```python
from build123d import *

# Parameters (mm, degrees)
SKETCH1_W                  = 25.4
SKETCH1_H                  = 1498.6
BOSS_EXTRUDE1_DEPTH        = 25.4
SKETCH2_W                  = 23.114
SKETCH2_H                  = 23.114
CUT_EXTRUDE1_DEPTH         = 1499.6
M3_5_CLEARANCE_HOLE1_D     = 4.1402
M3_5_CLEARANCE_HOLE1_DEPTH = 25.4
M3_5_CLEARANCE_HOLE2_D     = 4.1402
M3_5_CLEARANCE_HOLE2_DEPTH = 25.4
CHAMFER1_SIZE              = 2.159
FILLET1_R                  = 0.8128
FILLET2_R                  = 3.0988
SKETCH8_W                  = 95.882963774
SKETCH8_H                  = 79.338329604
CUT_EXTRUDE3_DEPTH         = 1371.6
SKETCH11_W                 = 51.462522779
SKETCH11_H                 = 66.676735099
CUT_EXTRUDE6_DEPTH         = 2.286


with BuildPart() as part:
    # Sketch1 → Boss-Extrude1 (new body)
    with BuildSketch(Plane(origin=(0, 0, 0), x_dir=(0, -1, 0), z_dir=(-1, 0, 0))):
        with Locations((-12.7, 0)):
            Rectangle(SKETCH1_W, SKETCH1_H)
    extrude(amount=-BOSS_EXTRUDE1_DEPTH)

    # Sketch2 → Cut-Extrude1 (cut, through all)
    with BuildSketch(Plane(origin=(0, 0, -749.3), x_dir=(-1, 0, 0), z_dir=(0, 0, -1))):
        with Locations((-13.843, 13.843)):
            Rectangle(SKETCH2_W, SKETCH2_H)
    extrude(amount=-CUT_EXTRUDE1_DEPTH, mode=Mode.SUBTRACT)

    # M3.5 Clearance Hole1
    with Locations(Plane(origin=(0, 0, 0), x_dir=(-1, 0, 0), z_dir=(0, -1, 0))):
        with Locations((-12.7, 736.6), (-12.7, 711.2), (-12.7, 685.8), (-12.7, 660.4), (-12.7, 635), (-12.7, 609.6), (-12.7, 584.2), (-12.7, 558.8), (-12.7, 533.4), (-12.7, 508), (-12.7, 482.6), (-12.7, 457.2), (-12.7, 431.8), (-12.7, 406.4), (-12.7, 381), (-12.7, 355.6), (-12.7, 330.2), (-12.7, 304.8), (-12.7, 279.4), (-12.7, 254), (-12.7, 228.6), (-12.7, 203.2), (-12.7, 177.8), (-12.7, 152.4), (-12.7, 127), (-12.7, 101.6), (-12.7, 76.2), (-12.7, 50.8), (-12.7, 25.4), (-12.7, 0), (-12.7, -25.4), (-12.7, -50.8), (-12.7, -76.2), (-12.7, -101.6), (-12.7, -127), (-12.7, -152.4), (-12.7, -177.8), (-12.7, -203.2), (-12.7, -228.6), (-12.7, -254), (-12.7, -279.4), (-12.7, -304.8), (-12.7, -330.2), (-12.7, -355.6), (-12.7, -381), (-12.7, -406.4), (-12.7, -431.8), (-12.7, -457.2), (-12.7, -482.6), (-12.7, -508), (-12.7, -533.4), (-12.7, -558.8), (-12.7, -584.2), (-12.7, -609.6), (-12.7, -635), (-12.7, -660.4), (-12.7, -685.8), (-12.7, -711.2), (-12.7, -736.6)):
            Hole(M3_5_CLEARANCE_HOLE1_D / 2, depth=M3_5_CLEARANCE_HOLE1_DEPTH)

    # M3.5 Clearance Hole2
    with Locations(Plane.ZY):
        with Locations((711.2, 12.7), (736.6, 12.7), (685.8, 12.7), (660.4, 12.7), (635, 12.7), (609.6, 12.7), (584.2, 12.7), (558.8, 12.7), (533.4, 12.7), (508, 12.7), (482.6, 12.7), (457.2, 12.7), (431.8, 12.7), (406.4, 12.7), (381, 12.7), (355.6, 12.7), (330.2, 12.7), (304.8, 12.7), (279.4, 12.7), (254, 12.7), (228.6, 12.7), (203.2, 12.7), (177.8, 12.7), (152.4, 12.7), (127, 12.7), (101.6, 12.7), (76.2, 12.7), (50.8, 12.7), (25.4, 12.7), (0, 12.7), (-25.4, 12.7), (-50.8, 12.7), (-76.2, 12.7), (-101.6, 12.7), (-127, 12.7), (-152.4, 12.7), (-177.8, 12.7), (-203.2, 12.7), (-228.6, 12.7), (-254, 12.7), (-279.4, 12.7), (-304.8, 12.7), (-330.2, 12.7), (-355.6, 12.7), (-381, 12.7), (-406.4, 12.7), (-431.8, 12.7), (-457.2, 12.7), (-482.6, 12.7), (-508, 12.7), (-533.4, 12.7), (-558.8, 12.7), (-584.2, 12.7), (-609.6, 12.7), (-635, 12.7), (-660.4, 12.7), (-685.8, 12.7), (-711.2, 12.7), (-736.6, 12.7)):
            Hole(M3_5_CLEARANCE_HOLE2_D / 2, depth=M3_5_CLEARANCE_HOLE2_DEPTH)

    # Chamfer1
    chamfer1_edges = [part.edges().sort_by_distance(p)[0] for p in [
        (25.4, 1.143, -749.3),
        (1.143, 25.4, 749.3),
        (1.143, 25.4, -749.3),
        (25.4, 1.143, 749.3),
    ]]
    chamfer(chamfer1_edges, length=CHAMFER1_SIZE)

    # Fillet1
    fillet1_edges = [part.edges().sort_by_distance(p)[0] for p in [
        (2.286, 2.286, 0),
    ]]
    fillet(fillet1_edges, radius=FILLET1_R)

    # Fillet2
    fillet2_edges = [part.edges().sort_by_distance(p)[0] for p in [
        (0, 0, 0),
    ]]
    fillet(fillet2_edges, radius=FILLET2_R)

    # Sketch8 → Cut-Extrude3 (cut)
    with BuildSketch(Plane.XY.offset(749.3)):
        with Locations((2.286, 3.0988)):
            Rectangle(SKETCH8_W, SKETCH8_H)
    extrude(amount=-CUT_EXTRUDE3_DEPTH, mode=Mode.SUBTRACT)

    # Sketch11 → Cut-Extrude6 (cut)
    with BuildSketch(Plane.XY.offset(-622.3)):
        with Locations((1.85517497, 1.74884985)):
            Rectangle(SKETCH11_W, SKETCH11_H)
    extrude(amount=-CUT_EXTRUDE6_DEPTH, mode=Mode.SUBTRACT)


solid = part.part
```
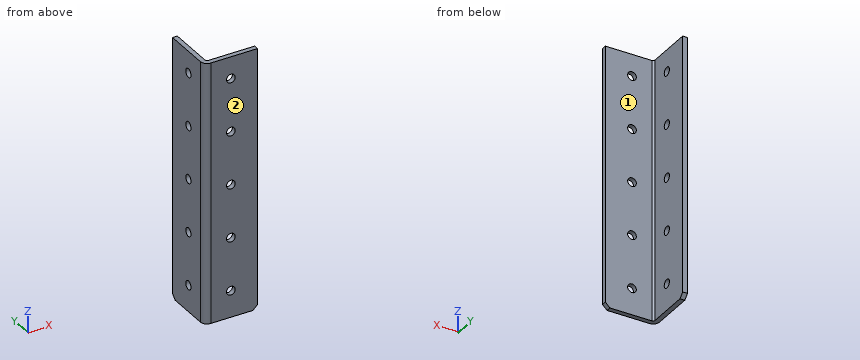
Read the model definition and answer for the solid it produces. Units are mm, in the model's axes. Face numbers are marked on the shaded views. A direction names the side the tool comes from. Give positions to 0.01 mm unless a question says otherwise; leave off trailing zeros. Write each loop counter-clockwise with the first axis right and the second up, starting at its lowest first coordinate (ties: lowest second). Pieces come first, ordered by that corner, then holes. Notation, with made-up numbers: M 54,9 L 81,9 A34 ccw 81,46 Z; hole C 56.25,-18 d8. An arc over 180 degrees is marked long. Put each result on its own line as item: value. Start each with the question number.
1. Which of the six approach directions +Z, -Z, +X, -X, +Y, -Y give full straight-line access (tool end or side, diameter ignored) to the marked faces 1 and 2?
2. The part is cut by section A-A, the plane z = -685.8. Give the vertices of the cut face in (x, y).
3. The part is cut by section C-C, the plane y = 4.5. Give the vertices of the cut face in (x, z), and give its area (3 significant figures).
4. Each of these flat-tipped pins is pushed along its axis until it touches: pin 1 Ø5.5 at (x, z) = (12.7, -660.4) entering from -Y; pin 2 Ø2 at (x, z) = (4, -677) entering from +Y; pin 3 Ø6.5 at (y, z) = (12.7, -711.2) entering from +X. Where does it stop, or does it pass through?
5. The part is cut by section B-B, the plane x = 12.7. Give the vertices of the cut face in (y, z), and give its area (3 significant figures).
6. Consider line 1 along Z through (x, y) = (12.7, 0.85); line 2 along X through (y, z) = (6, -631); line 3 along X through (y, z) = (0.7, -635). Determine where each line is inside the solid, lowest interval first.
Final values:
1. face 1: +Z, -Z, +X, +Y
1. face 2: +Z, -Z, +X, -X, -Y
2. outline: M 0,3.1 A3.1 ccw 3.1,0 L 10.63,0 L 10.63,2.29 L 3.1,2.29 A0.81 cw 2.29,3.1 L 2.29,10.63 L 0,10.63 Z; M 0,14.77 L 2.29,14.77 L 2.29,25.4 L 0,25.4 Z; M 14.77,0 L 25.4,0 L 25.4,2.29 L 14.77,2.29 Z
3. outline: M 0,-749.3 L 2.29,-749.3 L 2.29,-624.59 L 0,-624.59 Z
3. area: 285 mm²
4. pin 1: stops at y = 0
4. pin 2: stops at y = 2.29
4. pin 3: stops at x = 2.29
5. outline: M 0,-749.3 L 2.29,-749.3 L 2.29,-738.67 L 0,-738.67 Z; M 0,-734.53 L 2.29,-734.53 L 2.29,-713.27 L 0,-713.27 Z; M 0,-709.13 L 2.29,-709.13 L 2.29,-687.87 L 0,-687.87 Z; M 0,-683.73 L 2.29,-683.73 L 2.29,-662.47 L 0,-662.47 Z; M 0,-658.33 L 2.29,-658.33 L 2.29,-637.07 L 0,-637.07 Z; M 0,-632.93 L 2.29,-632.93 L 2.29,-624.59 L 0,-624.59 Z
5. area: 238 mm²
6. line 1: z = -749.3 to -738.67, -734.53 to -713.27, -709.13 to -687.87, -683.73 to -662.47, -658.33 to -637.07, -632.93 to -624.59
6. line 2: x = 0 to 2.29
6. line 3: x = 1.14 to 10.63, 14.77 to 25.4
